Check sheet for the modelled part. Datum: model origin and axes. Units: mm. A direction names the side the tool comes from. Coordinates: 2 decimals unless noted, no trailing zeros. Write each loop counter-clockwise with the first axis right and the second up, starting at its lowest first coordinate (ties: lowest second). Pieces come first, ordered by that corner, then holes. Notation, with made-up numbers: (55, -13) -> (66, -13) arc R29 ccw to (66, 23) -> close; hole circle Ø4 at (-13.5, -18). An arc over 180 degrees is marked (long way). One line per item, written item: value. Start each with the question number.
1) Draft check along Z on faces 1 (the cylindrical face through (-8.216, 2.958, 4.115)), 2 (the cylindrical face through (0.06, 2.55, 11.2)), 3 (the flat face through (-0.1, 4.4, 0)). Enter one of: +Z half, -Z half, draft (parallel to the pull), parting line (faces both ways), or undercut.
2) Sectioned sample at D-D on z = 10. Enter the section's corners in (x, y), plus the area to 3 significant figures.
3) Set-up check for faces 4 (the flat face through (0, 3, 7.5)), 5 (the cylindrical face through (4.19, 2.96, 11)), 6 (the flat face through (8.5, 3, 12)), 7 (the flat face through (0, 6, 7)), 8 (the flat face through (-8.5, 3, 12)): record each of +Z, -Z, +X, -X, +Y, -Y from which the full face is reachable in a straight line by a thin tool's end or side.
4) Gauge pin test, flat ends, axial feed: P1, Ø3, axis at x = 5.5, z = 12, coming from the -Y side; P2, Ø1.8, axis at y = 3.5, z = 11.5, coming from the -X side. Record the tip position at first contact, or that the pin passes through.
5) Sectioned sample at C-C on x = 0. Enter the section's corners in (y, z), plus the area to 3 significant figures.
6) Sectioned sample at B-B on y = 2. Give the number of separate pieces and of enclosed holes in the cut face, plus the area to 3 significant figures.
7) Sectioned sample at A-A on z = 3. Enter the section's corners in (x, y).
8) Scan lines: line 1 along Z through (x, y) = (7, 2.5); line 2 along X through (y, z) = (2, 11.75); line 3 along Z through (x, y) = (-6.5, 5). Record each from-to range of solid material in increasing order. Write a range as [from, to].
```python
from build123d import *

# Parameters (mm, degrees)
PAD_DEPTH       = 15
SKETCH003_W     = 20
SKETCH003_H     = 6
PAD001_DEPTH    = 7.5
SKETCH001_R     = 1.65
POCKET_DEPTH    = 6.001
SKETCH002_R     = 4.05
POCKET001_DEPTH = 7.5
CHAMFER_SIZE    = 1.49


with BuildPart() as part:
    # Sketch → Pad (new body)
    with BuildSketch(Plane.XY):
        with BuildLine():
            ThreePointArc((2.55, 0), (0, 2.55), (-2.55, 0))
            Line((-2.55, 0), (-8.5, 0))
            Line((-8.5, 0), (-8.5, 6))
            Line((-8.5, 6), (8.5, 6))
            Line((8.5, 6), (8.5, 0))
            Line((2.55, 0), (8.5, 0))
        make_face()
    extrude(amount=PAD_DEPTH)

    # Sketch003 → Pad001 (join)
    with BuildSketch(Plane.XY):
        with Locations((0, 3)):
            Rectangle(SKETCH003_W, SKETCH003_H)
    extrude(amount=PAD001_DEPTH)

    # Sketch001 → Pocket (cut, through all)
    with BuildSketch(Plane.XZ):
        with Locations((-7, 3)):
            Circle(SKETCH001_R)
        with Locations((-5.5, 12)):
            Circle(SKETCH001_R)
        with Locations((5.5, 12)):
            Circle(SKETCH001_R)
        with Locations((7, 3)):
            Circle(SKETCH001_R)
    extrude(amount=-POCKET_DEPTH, mode=Mode.SUBTRACT)

    # Sketch002 → Pocket001 (cut)
    with BuildSketch(Plane.XY):
        Circle(SKETCH002_R)
    extrude(amount=POCKET001_DEPTH, mode=Mode.SUBTRACT)

    # Chamfer
    chamfer_edges = [part.edges().sort_by_distance(p)[0] for p in [
        (8.5, 3, 7.5),
        (-8.5, 3, 7.5),
    ]]
    chamfer(chamfer_edges, length=CHAMFER_SIZE)


solid = part.part
```
Answers:
1. face 1: undercut
1. face 2: draft
1. face 3: -Z half
2. outline: (-8.5, 0) -> (-2.55, 0) arc R2.55 cw to (2.55, 0) -> (8.5, 0) -> (8.5, 6) -> (-8.5, 6) -> close
2. area: 91.8 mm2
3. face 4: -Z, -Y
3. face 5: +Y, -Y
3. face 6: +Z, +X, +Y, -Y
3. face 7: +Z, -Z, +X, -X, +Y
3. face 8: +Z, -X, +Y, -Y
4. P1: passes through
4. P2: stops at x = -8.5
5. outline: (2.55, 7.5) -> (4.05, 7.5) -> (4.05, 0) -> (6, 0) -> (6, 15) -> (2.55, 15) -> close
5. area: 40.5 mm2
6. separate pieces: 2
6. enclosed holes: 4
6. area: 169 mm2
7. outline: (-10, 0) -> (-8.65, 0) -> (-8.65, 6) -> (-10, 6) -> close; (-5.35, 0) -> (-4.05, 0) arc R4.05 cw to (4.05, 0) -> (5.35, 0) -> (5.35, 6) -> (-5.35, 6) -> close; (8.65, 0) -> (10, 0) -> (10, 6) -> (8.65, 6) -> close
8. line 1: z = [0, 1.35], [4.65, 11.31], [12.69, 15]
8. line 2: x = [-8.5, -7.13], [-3.87, -1.58], [1.58, 3.87], [7.13, 8.5]
8. line 3: z = [0, 1.43], [4.57, 10.69], [13.31, 15]
